```python
from build123d import *

# Parameters (mm, degrees)
SKETCH_1_W          = 75
SKETCH_1_H          = 45
SKETCH_1_R          = 2.65
EXTRUDE_1_DEPTH     = 3
SKETCH_2_W          = 20
SKETCH_2_H          = 45
EXTRUDE_2_DEPTH     = 3
SKETCH_3_R          = 1.6
CUT_EXTRUDE_1_DEPTH = 3
SKETCH_4_W          = 20
SKETCH_4_H          = 45
EXTRUDE_3_DEPTH     = 3


with BuildPart() as part:
    # 草图1 → 凸台-拉伸1 (new body)
    with BuildSketch(Plane.XY):
        with Locations((-219.5, 22.5)):
            Rectangle(SKETCH_1_W, SKETCH_1_H)
        with Locations((-239.5, 10)):
            Circle(SKETCH_1_R, mode=Mode.SUBTRACT)
        with Locations(Location((-199.5, 10, 0), (0, 0, 180))):
            Circle(SKETCH_1_R, mode=Mode.SUBTRACT)
    extrude(amount=EXTRUDE_1_DEPTH)

    # 草图2 → 凸台-拉伸2 (add)
    with BuildSketch(Plane.XY.offset(3)):
        with Locations((-172, 22.5)):
            Rectangle(SKETCH_2_W, SKETCH_2_H)
    extrude(amount=-EXTRUDE_2_DEPTH)

    # 草图3 → 切除-拉伸1 (cut)
    with BuildSketch(Plane.XY.offset(3)):
        with Locations((-197, 39)):
            Circle(SKETCH_3_R)
        with Locations((-177, 39)):
            Circle(SKETCH_3_R)
        with Locations((-232, 39)):
            Circle(SKETCH_3_R)
        with Locations((-252, 39)):
            Circle(SKETCH_3_R)
    extrude(amount=-CUT_EXTRUDE_1_DEPTH, mode=Mode.SUBTRACT)

    # 草图4 → 凸台-拉伸3 (add)
    with BuildSketch(Plane.XY.offset(3)):
        with Locations((-267, 22.5)):
            Rectangle(SKETCH_4_W, SKETCH_4_H)
    extrude(amount=-EXTRUDE_3_DEPTH)


solid = part.part
```
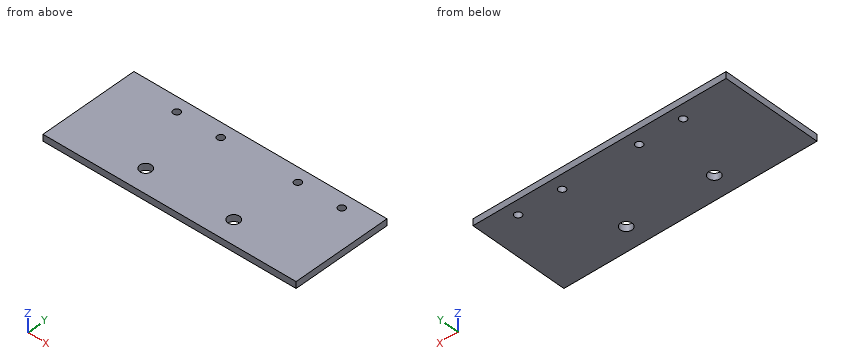
Can you work these out from the model? Positions are in its coordinate system, mm. Coordinates: 2 decimals unless noted, no trailing zeros. Loops run counter-clockwise (first coordinate to the right, second up) from the corner with the lowest first, then second, coordinate; pieces in that order, holes last.
1) I need wall thicknesses on probe 1 along Y at (x, z) = (-199.5, 1.9); probe 2 along X at (y, z) = (11, 2.15); probe 3 along Y at (x, z) = (-232, 1.4). Which ranges of each line are inside material? Lowest first, please.
2) For pin 1 (3 mm diameter, centred on x = -232, y = 39, fed in from +Z), with a flat end and sliding along its axis, tell me the tip position at first contact or that it passes through.
3) Imagine slicing it at B-B on y = 10. List the corners of the cut face in (x, z) for me, plus the area to 3 significant figures.
4) Imagine slicing it at C-C on y = 39. List the corners of the cut face in (x, z) for me.
5) Imagine slicing it at A-A on x = -232. List the corners of the cut face in (y, z) for me.
Completed:
1. probe 1: y = 0 to 7.35, 12.65 to 45
1. probe 2: x = -277 to -241.95, -237.05 to -201.95, -197.05 to -162
1. probe 3: y = 0 to 37.4, 40.6 to 45
2. pin 1: passes through
3. outline: (-277, 0) - (-242.15, 0) - (-242.15, 3) - (-277, 3) - close; (-236.85, 0) - (-202.15, 0) - (-202.15, 3) - (-236.85, 3) - close; (-196.85, 0) - (-162, 0) - (-162, 3) - (-196.85, 3) - close
3. area: 313 mm2
4. outline: (-277, 0) - (-253.6, 0) - (-253.6, 3) - (-277, 3) - close; (-250.4, 0) - (-233.6, 0) - (-233.6, 3) - (-250.4, 3) - close; (-230.4, 0) - (-198.6, 0) - (-198.6, 3) - (-230.4, 3) - close; (-195.4, 0) - (-178.6, 0) - (-178.6, 3) - (-195.4, 3) - close; (-175.4, 0) - (-162, 0) - (-162, 3) - (-175.4, 3) - close
5. outline: (0, 0) - (37.4, 0) - (37.4, 3) - (0, 3) - close; (40.6, 0) - (45, 0) - (45, 3) - (40.6, 3) - close
